Source: CAD feature listing. Evaluate the final solid. Frame: model axes, mm. A direction names the side the tool comes from. Coordinates: 2 decimals unless noted, no trailing zeros. Loops run counter-clockwise (first coordinate to the right, second up) from the corner with the lowest first, then second, coordinate; pieces in that order, holes last. Notation, with made-up numbers: M 14.5,12 L 18.5,12 A17 cw 18.5,21 Z; hole C 51.25,27.5 d10. An arc over 180 degrees is marked long. One line per question, with ' | ' between items. Start each with the question number.
1. Section query D-D, the plane y = 18.5. Output: boundary loops of the cut face in (x, z), and give its area (3 significant figures).
2. Section query C-C, the plane y = -12. Output: boundary loops of the cut face in (x, z), and give its area (3 significant figures).
3. Pin query (flat end, axial travel): P1, Ø6.5, axis at y = -3.5, z = 8, coming from the -X side; P2, Ø3, axis at y = 10.5, z = 4, coming from the -X side; P3, Ø4, axis at x = -15.5, z = 9, coming from the +Y side. Return the tip coordinate at first contact, or that it passes through.
4. Access query for faces 1 (the flat face through (-15, 16, 0)), 2 (the flat face through (-25, -17.014, 6)). Directions: +Z, -Z, +X, -X, +Y, -Y. A direction counts if a zero-diameter tool reaches every point of the face in a straight line with its end or side. Return the directions, or none.
5. Mould query, pull axis X, two halves, no side actions, for faces 3 (the cylindrical face through (-67.63, -1.36, 6.26)), 4 (the flat face through (24.753, -2, 6)), 5 (the flat face through (0, -1, 6)), 6 (the flat face through (-11, 23.109, 6)). Classes: pulls with the +X half, pulls with the -X half, needs draft (parallel to the pull), parting line crosses it, or undercut.
6. Ray query, probe 1 along Y at (x, z) = (-29, 1.5); probe 2 along X at (y, z) = (-0.5, 5); probe 3 along Y at (x, z) = (7, 11.5). Return the intervals inside material, ascending.
7. Section query B-B, the plane z = 11.25. Output: boundary loops of the cut face in (x, y), and give its area (3 significant figures).
8. Section query A-A, the plane x = -41.5. Output: boundary loops of the cut face in (y, z), and give its area (3 significant figures).
```python
from build123d import *

# Parameters (mm, degrees)
F1_DEPTH = 12.7


with BuildPart() as f1:
    # F0 (on Top) → F1 (new body)
    with BuildSketch(Plane.XY):
        with BuildLine():
            ThreePointArc((-47.3058475157, 23.1087561697), (-76.0328855481, 1.1598869775), (-51.6270473599, -25.511270389))
            Line((-51.6270473599, -25.511270389), (-51.6270473599, -17.0142557472))
            ThreePointArc((-51.6270473599, -17.0142557472), (-67.6320735365, -1.0092295706), (-51.6270473599, 14.9957966059))
            Line((-51.6270473599, 14.9957966059), (-51.6270473599, 23.1087561697))
            Line((-51.6270473599, 23.1087561697), (-47.3058475157, 23.1087561697))
        make_face()
        with BuildLine():
            ThreePointArc((-33.0747121606, -17.0142557472), (-41.4242487344, -23.2859641713), (-51.6270473599, -25.511270389))
            Line((-51.6270473599, -25.511270389), (24.7534979135, -25.511270389))
            Line((24.7534979135, -25.511270389), (24.7534979135, 23.1087561697))
            Line((24.7534979135, 23.1087561697), (-47.3058475157, 23.1087561697))
            ThreePointArc((-47.3058475157, 23.1087561697), (-39.4921934437, 20.2768063378), (-33.0747121606, 14.9957966059))
            Line((-33.0747121606, 14.9957966059), (0, 14.9957966059))
            Line((0, 14.9957966059), (0, -17.0142557472))
            Line((0, -17.0142557472), (-33.0747121606, -17.0142557472))
        make_face()
        with BuildLine():
            Line((-51.6270473599, -17.0142557472), (-51.6270473599, -25.511270389))
            ThreePointArc((-51.6270473599, -25.511270389), (-41.4242487344, -23.2859641713), (-33.0747121606, -17.0142557472))
            Line((-33.0747121606, -17.0142557472), (-51.6270473599, -17.0142557472))
        make_face()
        with BuildLine():
            ThreePointArc((-33.0747121606, 14.9957966059), (-39.4921934437, 20.2768063378), (-47.3058475157, 23.1087561697))
            Line((-47.3058475157, 23.1087561697), (-51.6270473599, 23.1087561697))
            Line((-51.6270473599, 23.1087561697), (-51.6270473599, 14.9957966059))
            Line((-51.6270473599, 14.9957966059), (-33.0747121606, 14.9957966059))
        make_face()
    extrude(amount=F1_DEPTH)


solid = f1.part
```
Taken from the geometry:
1) outline: M -66.45,0 L 24.75,0 L 24.75,12.7 L -66.45,12.7 Z | area: 1,160 mm^2
2) outline: M -73.53,0 L -63.26,0 L -63.26,12.7 L -73.53,12.7 Z; M 0,0 L 24.75,0 L 24.75,12.7 L 0,12.7 Z | area: 445 mm^2
3) P1: x = -76.13 | P2: x = -73.99 | P3: y = 23.11
4) face 1: -Z, +X, -X, +Y, -Y | face 2: +Z, -Z
5) face 3: undercut | face 4: pulls with the +X half | face 5: undercut | face 6: needs draft
6) probe 1: -25.51 to -17.01, 15 to 23.11 | probe 2: -76.12 to -67.62, 0 to 24.75 | probe 3: -25.51 to 23.11
7) outline: M -51.63,-25.51 L 24.75,-25.51 L 24.75,23.11 L -47.31,23.11 A24.5 ccw long Z; hole M -51.63,-17.01 L 0,-17.01 L 0,15 L -51.63,15 A16.01 ccw Z | area: 2,600 mm^2
8) outline: M -25.51,0 L -17.01,0 L -17.01,12.7 L -25.51,12.7 Z; M 15,0 L 23.11,0 L 23.11,12.7 L 15,12.7 Z | area: 211 mm^2
